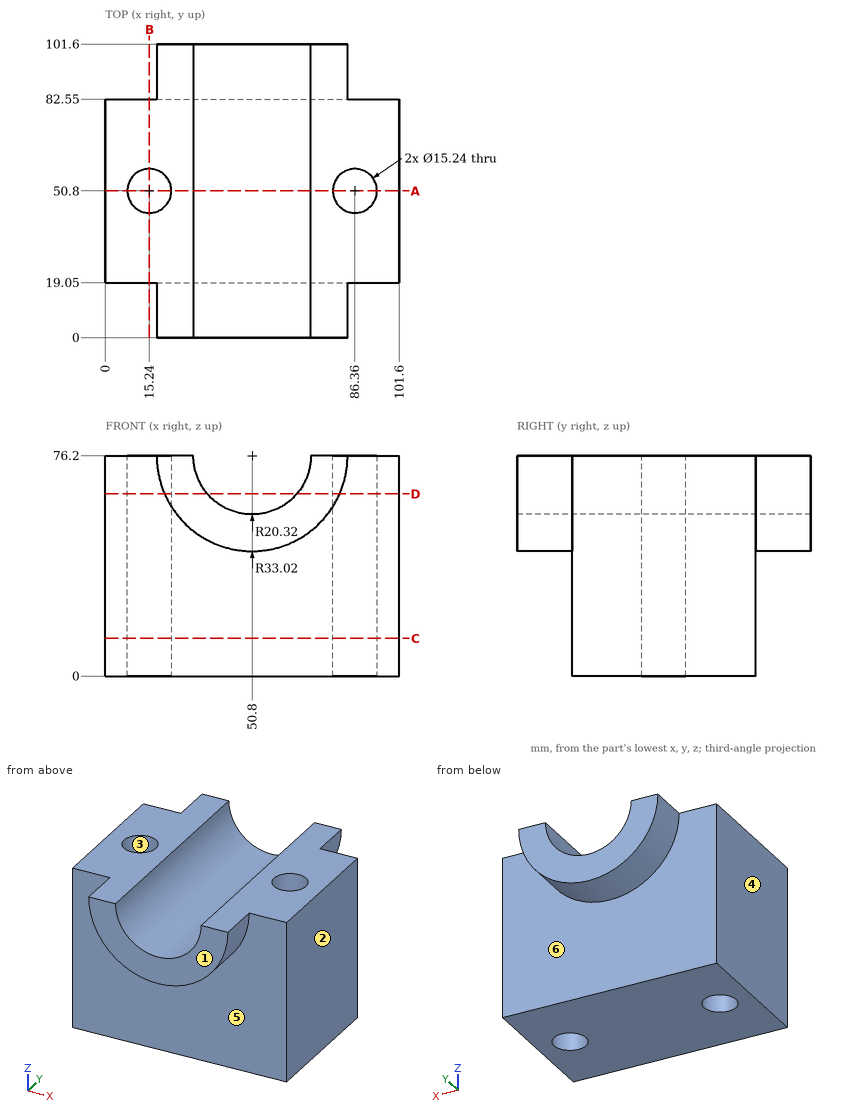
Print and shaded views of the part. All mm, measured from the part's lowest x, y and z. A direction names the side the tool comes from. Coordinates: 2 decimals unless noted, no trailing zeros. Order: outer loops, then holes, each group sorted by start corner. A loop starts at its lowest first (then second) coordinate and runs counter-clockwise, first axis right, second up. Notation, with made-up numbers: (51, 73.5) -> (92, 73.5) arc R26 cw to (92, 107.5) -> close; hole circle Ø1 at (38, -1.5). An arc over 180 degrees is marked (long way). Use one line per item in the form item = value. Start each with the question number.
1) Band-saw the part on B-B on x = 15.24. Give the cut face in (y, z), then the cut area to 3 significant figures.
2) Drill centre lines: L1, parallel to Y at x = 86, z = 35; L2, parallel to X at y = 50, z = 32; L3, parallel to X at y = 21, z = 67.5. Where is each one in solid material? Low to high. Write a range as [from, to].
3) Band-saw the part on D-D on z = 63. Give the cut face in (x, y).
4) Band-saw the part on A-A on y = 50.8. Give the cut face in (x, z), then the cut area to 3 significant figures.
5) Pull direction Y, two halves, no side cores. Call the marked faces 1, 2 and 3: +Y half, -Y half, draft (parallel to the pull), parting line (faces both ways), or undercut.
6) Band-saw the part on C-C on z = 13. Give the cut face in (x, y).
7) Drop flat-ended pins along their axis: pin 1 (4 mm diameter, centred on x = 15, z = 10.5, fed in from +Y); pin 2 (17.5 mm diameter, centred on x = 15.24, y = 50.8, fed in from -Z); pin 3 (10 mm diameter, centred on x = 17, z = 41.5, fed in from -Y). Give the stop position or say it passes through.
8) Tool access for the marked faces 4, 5 and 6: list every direction of +Z, -Z, +X, -X, +Y, -Y with a clear straight run to the whole face (end or side of a thin tool).
Entries:
q1.outline = (19.05, 0) -> (43.18, 0) -> (43.18, 76.2) -> (19.05, 76.2) -> close; (58.42, 0) -> (82.55, 0) -> (82.55, 76.2) -> (58.42, 76.2) -> close
q1.area = 3,680 mm2
q2.L1 = [19.05, 43.19], [58.41, 82.55]
q2.L2 = [0, 7.66], [22.82, 78.78], [93.94, 101.6]
q2.L3 = [0, 32.44], [69.16, 101.6]
q3.outline = (0, 19.05) -> (20.53, 19.05) -> (20.53, 0) -> (35.35, 0) -> (35.35, 101.6) -> (20.53, 101.6) -> (20.53, 82.55) -> (0, 82.55) -> close; (66.25, 0) -> (81.07, 0) -> (81.07, 19.05) -> (101.6, 19.05) -> (101.6, 82.55) -> (81.07, 82.55) -> (81.07, 101.6) -> (66.25, 101.6) -> close; hole circle Ø15.24 at (15.24, 50.8); hole circle Ø15.24 at (86.36, 50.8)
q4.outline = (0, 0) -> (7.62, 0) -> (7.62, 76.2) -> (0, 76.2) -> close; (22.86, 0) -> (78.74, 0) -> (78.74, 76.2) -> (71.12, 76.2) arc R20.32 cw to (30.48, 76.2) -> (22.86, 76.2) -> close; (93.98, 0) -> (101.6, 0) -> (101.6, 76.2) -> (93.98, 76.2) -> close
q4.area = 4,770 mm2
q5.face_1 = -Y half
q5.face_2 = draft
q5.face_3 = undercut
q6.outline = (0, 19.05) -> (101.6, 19.05) -> (101.6, 82.55) -> (0, 82.55) -> close; hole circle Ø15.24 at (15.24, 50.8); hole circle Ø15.24 at (86.36, 50.8)
q7.pin_1 = 82.55
q7.pin_2 = 0
q7.pin_3 = 19.05
q8.face_4 = +Z, -Z, -X, +Y, -Y
q8.face_5 = -Z, -Y
q8.face_6 = -Z, +Y
